Design review of the part built by this model. Coordinates are the model's own, in mm. Face numbers are marked on the shaded views. A direction names the side the tool comes from. Round coordinates to 2 decimals unless told otherwise and drop trailing zeros. Order: outer loops, then holes, each group sorted by start corner. A loop starts at its lowest first (then second) coordinate and runs counter-clockwise, first axis right, second up. Notation, with made-up numbers: M 77.25,5.25 L 123.25,5.25 A21 ccw 123.25,29.25 Z; hole C 60.5,73 d4. An arc over 180 degrees is marked long. Use a Markdown table: item, result. Add a question column.
(1) Machinability: for the marked faces 1, 2, 3, 4 and 5, which of the approach directions +Z, -Z, +X, -X, +Y, -Y give a long, thin tool a straight path to every point of the face, cutting with its end or side? Answer none if there is none.
(2) Take a section at C-C (y = 13.7). Write out the cut boundary in (x, z).
(3) To check wall thickness, follow probe 1 along Y at (x, z) = (-8.5, 0.5); probe 2 along Z at (x, y) = (15.9, 0.4); probe 3 along Y at (x, z) = (0, 3.25). State the ranges of each line that lie inside material, in increasing order. Write a range as from..to.
(4) For pin 1 (2.5 mm diameter, centred on x = 9, z = 2.5, fed in from +Y); pin 2 (3 mm diameter, centred on x = -7.9, z = 3.95, fed in from -Y); pin 3 (2.5 mm diameter, centred on y = 10.5, z = 2, fed in from -X); pin 4 (2.5 mm diameter, centred on y = 12, z = 3, fed in from +X), all flat-tipped, find the tip position at first contact; note any pin that passes through.
(5) The part is to be moulded in two halves that separate along Y. For the marked faces 6, 7, 8 and 9, say which applies: released by +Y, released by -Y, zero draft, split by the parting line, or undercut.
(6) Take a section at A-A (x = 0). Write out the cut boundary in (y, z), then the cut area to 3 significant figures.
(7) Take a section at B-B (z = 6.75). Write out the cut boundary in (x, y).
(8) Take a section at D-D (x = -7.9). Write out the cut boundary in (y, z).
```python
from build123d import *

# Parameters (mm, degrees)
PAD_DEPTH       = 7.8
SKETCH001_R     = 1.55
POCKET_DEPTH    = 17.701
SKETCH002_R     = 1.55
POCKET001_DEPTH = 7.801


with BuildPart() as part:
    # Sketch → Pad (new body)
    with BuildSketch(Plane.XY):
        Polygon((-3.9, 17.7), (3.9, 17.7), (3.9, 7.8), (19.9, 7.8), (19.9, 6), (3.9, 6), (3.9, 1.8), (19.9, 1.8), (19.9, 0), (-19.9, 0), (-19.9, 1.8), (-3.9, 1.8), (-3.9, 6), (-19.9, 6), (-19.9, 7.8), (-3.9, 7.8), align=None)
    extrude(amount=PAD_DEPTH)

    # Sketch001 (on Face11 of Pad) → Pocket (cut, through all)
    with BuildSketch(Plane.XZ):
        with Locations((-15.9, 3.95)):
            Circle(SKETCH001_R)
        with Locations((-7.9, 3.95)):
            Circle(SKETCH001_R)
        with Locations((7.9, 3.95)):
            Circle(SKETCH001_R)
        with Locations((15.9, 3.95)):
            Circle(SKETCH001_R)
    extrude(amount=-POCKET_DEPTH, mode=Mode.SUBTRACT)

    # Sketch002 (on Face4 of Pocket) → Pocket001 (cut, through all)
    with BuildSketch(Plane.XY.offset(7.8)):
        with Locations((0, 13.7)):
            Circle(SKETCH002_R)
    extrude(amount=-POCKET001_DEPTH, mode=Mode.SUBTRACT)


solid = part.part
```
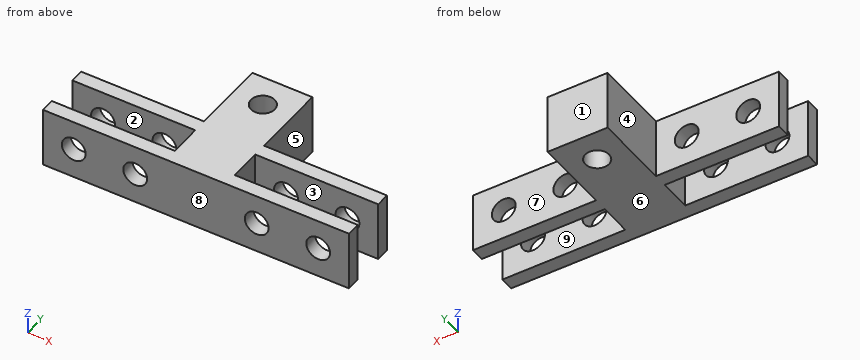
Verdict:
| question | item | result |
|---|---|---|
| 1 | face 1 | +Z, -Z, +X, -X, +Y |
| 1 | face 2 | +Z, -Z, -X |
| 1 | face 3 | +Z, -Z, +X |
| 1 | face 4 | +Z, -Z, -X, +Y |
| 1 | face 5 | +Z, -Z, +X, +Y |
| 2 | outline | M -3.9,0 L -1.55,0 L -1.55,7.8 L -3.9,7.8 Z; M 1.55,0 L 3.9,0 L 3.9,7.8 L 1.55,7.8 Z |
| 3 | probe 1 | y = 0..1.8, 6..7.8 |
| 3 | probe 2 | z = 0..2.4, 5.5..7.8 |
| 3 | probe 3 | y = 0..12.15, 15.25..17.7 |
| 4 | pin 1 | stops at y = 7.8 |
| 4 | pin 2 | passes through |
| 4 | pin 3 | stops at x = -3.9 |
| 4 | pin 4 | stops at x = 3.9 |
| 5 | face 6 | zero draft |
| 5 | face 7 | released by +Y |
| 5 | face 8 | released by -Y |
| 5 | face 9 | undercut |
| 6 | outline | M 0,0 L 12.15,0 L 12.15,7.8 L 0,7.8 Z; M 15.25,0 L 17.7,0 L 17.7,7.8 L 15.25,7.8 Z |
| 6 | area | 114 mm^2 |
| 7 | outline | M -19.9,0 L 19.9,0 L 19.9,1.8 L 3.9,1.8 L 3.9,6 L 19.9,6 L 19.9,7.8 L 3.9,7.8 L 3.9,17.7 L -3.9,17.7 L -3.9,7.8 L -19.9,7.8 L -19.9,6 L -3.9,6 L -3.9,1.8 L -19.9,1.8 Z; hole C 0,13.7 d3.1 |
| 8 | outline | M 0,0 L 1.8,0 L 1.8,2.4 L 0,2.4 Z; M 0,5.5 L 1.8,5.5 L 1.8,7.8 L 0,7.8 Z; M 6,0 L 7.8,0 L 7.8,2.4 L 6,2.4 Z; M 6,5.5 L 7.8,5.5 L 7.8,7.8 L 6,7.8 Z |
